For this review, take the finished solid that the model builds, in its own axes (mm). Coordinates: 2 decimals unless noted, no trailing zeros. Write each loop counter-clockwise with the first axis right and the second up, starting at its lowest first coordinate (ties: lowest second). Pieces come first, ordered by that corner, then holes.
1) We need section A-A on z = 1.7. Give the number of separate pieces and of enclosed holes in the cut face, then the cut area to 3 significant figures.
2) Insertion check: P1, Ø1.5, axis at y = 49, z = 0.5, coming from the -X side; P2, Ø1.5, axis at x = -51, z = 2, coming from the +Y side; P3, Ø1.5, axis at y = -55.5, z = 1.5, coming from the +X side. Each pin has a flat end and moves straight along its axis. Give the tip position at first contact, or say it passes through.
3) We need section B-B on x = 63.5. Write out the cut boundary in (y, z).
4) To check wall thickness, follow line 1 along X through (y, z) = (-5, 1.2); line 2 along X through (y, z) = (28.5, 2.95); line 3 along X through (y, z) = (-39, 1.5). State the ranges of each line that lie inside material, in increasing order.
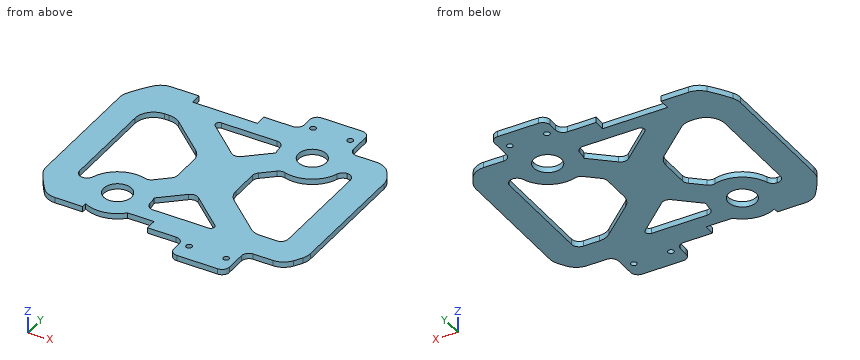
from build123d import *

# Parameters (mm, degrees)
ESBO_O1_R                = 7.5
ESBO_O1_R_2              = 1.6
RESSALTO_EXTRUS_O1_DEPTH = 3
FILETE2_R                = 10
FILETE3_R                = 4
FILETE4_R                = 2


with BuildPart() as part:
    # Esboço1 → Ressalto-extrusão1 (new body)
    with BuildSketch(Plane.XY):
        with BuildLine():
            Line((14.471901241, -53.5), (14.471901241, -66.5))
            Line((14.471901241, -66.5), (44.471901241, -66.5))
            Line((44.471901241, -66.5), (44.471901241, -47.5))
            Line((44.471901241, -47.5), (64.371965948, -47.5))
            ThreePointArc((64.371965948, -47.5), (68.06268346, -42.041302552), (71.291651246, -36.297389198))
            Line((71.291651246, -36.297389198), (71.291651246, 36.297389198))
            ThreePointArc((71.291651246, 36.297389198), (68.06268346, 42.041302552), (64.371965948, 47.5))
            Line((64.371965948, 47.5), (44.471901241, 47.5))
            Line((44.471901241, 47.5), (44.471901241, 66.5))
            Line((44.471901241, 66.5), (14.471901241, 66.5))
            Line((14.471901241, 66.5), (14.471901241, 53.5))
            Line((14.471901241, 53.5), (-5.003543323, 53.5))
            Line((-5.003543323, 53.5), (-5.003543323, 47.5))
            Line((-5.003543323, 47.5), (-40.003543323, 47.5))
            Line((-40.003543323, 47.5), (-40.003543323, 53.5))
            Line((-40.003543323, 53.5), (-59.478987886, 53.5))
            ThreePointArc((-59.478987886, 53.5), (-65.948635083, 45.285511266), (-71.291651246, 36.297389198))
            Line((-71.291651246, 36.297389198), (-71.291651246, -36.297389198))
            ThreePointArc((-71.291651246, -36.297389198), (-65.948635083, -45.285511266), (-59.478987886, -53.5))
            Line((-59.478987886, -53.5), (-40.003543323, -53.5))
            Line((-40.003543323, -53.5), (-40.003543323, -50.748788204))
            ThreePointArc((-40.003543323, -50.748788204), (-29.078718374, -52.589059769), (-19.237993286, -47.5))
            Line((-19.237993286, -47.5), (-5.003543323, -47.5))
            Line((-5.003543323, -47.5), (-5.003543323, -53.5))
            Line((-5.003543323, -53.5), (14.471901241, -53.5))
        make_face()
        with Locations((-31.783703802, -35.29937921)):
            Circle(ESBO_O1_R, mode=Mode.SUBTRACT)
        with Locations((19.471901241, -57)):
            Circle(ESBO_O1_R_2, mode=Mode.SUBTRACT)
        with Locations((39.471901241, -57)):
            Circle(ESBO_O1_R_2, mode=Mode.SUBTRACT)
        with BuildLine():
            Line((25, -39.332538239), (-14.754798134, -39.332538239))
            ThreePointArc((-14.754798134, -39.332538239), (-14.287636143, -34.928412284), (-14.941054623, -30.548045856))
            Line((-14.941054623, -30.548045856), (0, -17.5))
            Line((0, -17.5), (25, -39.332538239))
        make_face(mode=Mode.SUBTRACT)
        with BuildLine():
            Line((-15, -10.684767074), (-24.807750727, -19.249890785))
            ThreePointArc((-24.807750727, -19.249890785), (-40.174599446, -19.942202702), (-49.058352164, -32.5))
            Line((-49.058352164, -32.5), (-56.291651246, -32.5))
            Line((-56.291651246, -32.5), (-56.291651246, 32.5))
            Line((-56.291651246, 32.5), (-39.980184035, 32.5))
            Line((-39.980184035, 32.5), (-15, 10.684767074))
            Line((-15, 10.684767074), (-15, -10.684767074))
        make_face(mode=Mode.SUBTRACT)
        with BuildLine():
            Line((49.058352164, 32.5), (56.291651246, 32.5))
            Line((56.291651246, 32.5), (56.291651246, -32.5))
            Line((56.291651246, -32.5), (39.980184035, -32.5))
            Line((39.980184035, -32.5), (15, -10.684767074))
            Line((15, -10.684767074), (15, 10.684767074))
            Line((15, 10.684767074), (24.807750727, 19.249890785))
            ThreePointArc((24.807750727, 19.249890785), (40.174599446, 19.942202702), (49.058352164, 32.5))
        make_face(mode=Mode.SUBTRACT)
        with BuildLine():
            Line((0, 17.5), (-25, 39.332538239))
            Line((-25, 39.332538239), (14.754798134, 39.332538239))
            ThreePointArc((14.754798134, 39.332538239), (14.287636143, 34.928412284), (14.941054623, 30.548045856))
            Line((14.941054623, 30.548045856), (0, 17.5))
        make_face(mode=Mode.SUBTRACT)
        with Locations((19.471901241, 57)):
            Circle(ESBO_O1_R_2, mode=Mode.SUBTRACT)
        with Locations((39.471901241, 57)):
            Circle(ESBO_O1_R_2, mode=Mode.SUBTRACT)
        with Locations((31.783703802, 35.29937921)):
            Circle(ESBO_O1_R, mode=Mode.SUBTRACT)
    extrude(amount=RESSALTO_EXTRUS_O1_DEPTH)

    # Filete2
    filete2_edges = [part.edges().sort_by_distance(p)[0] for p in [
        (-15, 10.684767074, 1.5),
        (-39.980184035, 32.5, 1.5),
        (-56.291651246, 32.5, 1.5),
        (-59.478987886, -53.5, 1.5),
        (-71.291651246, -36.297389198, 1.5),
        (-71.291651246, 36.297389198, 1.5),
        (-59.478987886, 53.5, 1.5),
        (64.371965948, 47.5, 1.5),
        (71.291651246, 36.297389198, 1.5),
        (71.291651246, -36.297389198, 1.5),
        (64.371965948, -47.5, 1.5),
        (15, -10.684767074, 1.5),
        (39.980184035, -32.5, 1.5),
    ]]
    fillet(filete2_edges, radius=FILETE2_R)

    # Filete3
    filete3_edges = [part.edges().sort_by_distance(p)[0] for p in [
        (56.291651246, -32.5, 1.5),
        (56.291651246, 32.5, 1.5),
        (49.058352164, 32.5, 1.5),
        (24.807750727, 19.249890785, 1.5),
        (14.754798134, 39.332538239, 1.5),
        (0, 17.5, 1.5),
        (-15, -10.684767074, 1.5),
        (-56.291651246, -32.5, 1.5),
        (-49.058352164, -32.5, 1.5),
        (-24.807750727, -19.249890785, 1.5),
        (-14.754798134, -39.332538239, 1.5),
        (0, -17.5, 1.5),
        (14.471901241, 53.5, 1.5),
        (14.471901241, 66.5, 1.5),
        (44.471901241, 66.5, 1.5),
        (44.471901241, 47.5, 1.5),
        (44.471901241, -47.5, 1.5),
        (44.471901241, -66.5, 1.5),
        (14.471901241, -66.5, 1.5),
        (14.471901241, -53.5, 1.5),
        (15, 10.684767074, 1.5),
    ]]
    fillet(filete3_edges, radius=FILETE3_R)

    # Filete4
    filete4_edges = [part.edges().sort_by_distance(p)[0] for p in [
        (-25, 39.332538239, 1.5),
        (25, -39.332538239, 1.5),
    ]]
    fillet(filete4_edges, radius=FILETE4_R)


solid = part.part
Result:
1. separate pieces: 1
1. enclosed holes: 10
1. area: 9,900 mm2
2. P1: stops at x = -63.81
2. P2: stops at y = 53.5
2. P3: stops at x = 44.47
3. outline: (-46.48, 0) - (46.48, 0) - (46.48, 3) - (-46.48, 3) - close
4. line 1: x = -71.29 to -56.29, -15 to 15, 56.29 to 71.29
4. line 2: x = -71.29 to -54.29, -35.4 to -12.6, 12.6 to 28.62, 34.95 to 47.91, 56.29 to 71.29
4. line 3: x = -69.85 to -38.31, -25.26 to -11.88, 20.77 to 69.85
